Source: CAD feature listing. Evaluate the final solid. Frame: model axes, mm. A direction names the side the tool comes from. Round coordinates to 2 decimals unless told otherwise and drop trailing zeros. Order: outer loops, then holes, each group sorted by start corner. A loop starts at its lowest first (then second) coordinate and runs counter-clockwise, first axis right, second up. Notation, with made-up numbers: (-3, 16.25) - (35, 16.25) arc R5 ccw to (35, 21.25) - close; hole circle Ø9 at (-19.5, 46). An arc over 180 degrees is marked (long way). Return JSON: item names as keys, results as strings. Group by question number.
1) Ray query, line 1 (X direction, y = 4.5, z = 7.45); line 2 (Z direction, x = 12.7, y = 4.5); line 3 (X direction, y = 6.25, z = 19.5). Return the intervals inside material, ascending. Write a range as from..to.
2) Section C-C, the plane x = -2. Return loops of the section in (y, z).
3) Section A-A, the plane y = 8. Return loops of the section in (x, z).
4) Contact query for flat-ended pins moving along their axis: P1, Ø6, axis at y = 10, z = 29, coming from the -X side; P2, Ø6, axis at x = 1.5, z = 15, coming from the -Y side; P3, Ø1.5, axis at x = 12.7, z = 7.45, coming from the +Y side; P4, Ø3, axis at x = -12.7, z = 7.45, coming from the -Y side. Output: stop coordinate, or through.
5) Access query for faces 4 (the cylindrical face through (12.028, 5.916, 6.396)), 5 (the cylindrical face through (3.03, 3.52, 25.54)). Directions: +Z, -Z, +X, -X, +Y, -Y. A direction counts if a zero-diameter tool reaches every point of the face in a straight line with its end or side. Return the directions, or none.
6) Section B-B, the plane x = 12. Return loops of the section in (y, z), plus the area to 3 significant figures.
7) Section D-D, the plane z = 15.5. Return loops of the section in (x, y).
8) Mould query, pull axis Z, two halves, no side actions, for faces 1 (the flat face through (0, 6, 10.75)), 2 (the flat face through (0, 12, 0)), 3 (the cylindrical face through (-13.855, 5.916, 7.929)). Classes: pulls with the +Z half, pulls with the -Z half, needs draft (parallel to the pull), parting line crosses it, or undercut.
```python
from build123d import *

# Parameters (mm, degrees)
SKETCH_1_W         = 32
SKETCH_1_H         = 21.5
EXTRUDE_1_DEPTH    = 12
HOLE_WIZARD_M3_1_D = 2.5
FILLET_1_R         = 3
SKETCH_4_R         = 2.5
EXTRUDE_2_DEPTH    = 30


with BuildPart() as part:
    # 草图1 → 凸台-拉伸1 (new body)
    with BuildSketch(Plane(origin=(0, 0, 0), x_dir=(1, 0, 0), z_dir=(0, 1, 0))):
        Rectangle(SKETCH_1_W, SKETCH_1_H)
    extrude(amount=EXTRUDE_1_DEPTH)

    # M3 螺纹孔1 (through all)
    with Locations(Plane(origin=(0, 12, 0), x_dir=(1, 0, 0), z_dir=(0, 1, 0))):
        with Locations((-12.7, -7.45), (12.7, -7.45)):
            Hole(HOLE_WIZARD_M3_1_D / 2)

    # 圆角1
    fillet_1_edges = [part.edges().sort_by_distance(p)[0] for p in [
        (16, 6, 10.75),
        (-16, 6, 10.75),
    ]]
    fillet(fillet_1_edges, radius=FILLET_1_R)

    # 草图4 → 凸台-拉伸2 (add)
    with BuildSketch(Plane.XY.offset(10.75)):
        with Locations(Location((2.7, 6, 0), (0, 0, 180))):
            Circle(SKETCH_4_R)
    extrude(amount=EXTRUDE_2_DEPTH)


solid = part.part
```
Geometry check:
{
 "1": {"line 1": "-16..-13.95, -11.45..11.45, 13.95..16", "line 2": "-10.75..6.2, 8.7..10.75", "line 3": "0.21..5.19"},
 "2": {"outline": "(0, -10.75) - (12, -10.75) - (12, 10.75) - (0, 10.75) - close"},
 "3": {"outline": "(-16, -10.75) - (16, -10.75) - (16, 7.75) arc R3 ccw to (13, 10.75) - (4.2, 10.75) - (4.2, 40.75) - (1.2, 40.75) - (1.2, 10.75) - (-13, 10.75) arc R3 ccw to (-16, 7.75) - close; hole circle Ø2.5 at (-12.7, 7.45); hole circle Ø2.5 at (12.7, 7.45)"},
 "4": {"P1": "x = 0.41", "P2": "y = 3.5", "P3": "through", "P4": "y = 0"},
 "5": {"face 4": "+Y, -Y", "face 5": "+Z"},
 "6": {"outline": "(0, -10.75) - (12, -10.75) - (12, 6.41) - (0, 6.41) - close; (0, 8.49) - (12, 8.49) - (12, 10.75) - (0, 10.75) - close", "area": "233 mm2"},
 "7": {"outline": "circle Ø5 at (2.7, 6)"},
 "8": {"face 1": "pulls with the +Z half", "face 2": "needs draft", "face 3": "undercut"}
}
